from build123d import *

# Parameters (mm, degrees)
F0_W     = 134.5710605383
F0_H     = 126.8914490938
F0_W_2   = 120.110668242
F0_H_2   = 106.3882932067
F1_DEPTH = 50.8
F2_R     = 8.7009101407
F3_DEPTH = 508
F4_DEPTH = 25.4
F6_W     = 55.7228904217
F6_H     = 25.6094848633
F7_DEPTH = 584.2
F5_W     = 118.594430387
F5_H     = 112.178966403
F8_DEPTH = 508


with BuildPart() as f1:
    # F0 (on Top) → F1 (new body)
    with BuildSketch(Plane.XY):
        Rectangle(F0_W, F0_H)
        Rectangle(F0_W_2, F0_H_2, mode=Mode.SUBTRACT)
        Rectangle(F0_W_2, F0_H_2)
    extrude(amount=F1_DEPTH)

    # F2 (on face) → F3 (cut)
    with BuildSketch(Plane(origin=(-67.2855302691, 0, 0), x_dir=(0, -1, 0), z_dir=(-1, 0, 0))):
        with Locations((0, 22.9123719037)):
            Circle(F2_R)
    extrude(amount=-F3_DEPTH, mode=Mode.SUBTRACT)

    # F4 (add): a face of the model
    f4_faces = [f1.faces().sort_by_distance(p)[0] for p in [
        (0, 0, 50.8),
    ]]
    extrude(f4_faces, amount=F4_DEPTH)

    # F6 (on face) → F7 (cut)
    with BuildSketch(Plane(origin=(0, 63.4457245469, 0), x_dir=(-1, 0, 0), z_dir=(0, 1, 0))):
        with Locations((0.0916505232, 63.3952575684)):
            Rectangle(F6_W, F6_H)
    extrude(amount=-F7_DEPTH, mode=Mode.SUBTRACT)

    # F5 (on face) → F8 (cut)
    with BuildSketch(Plane.XY.offset(76.2)):
        Rectangle(F5_W, F5_H)
    extrude(amount=-F8_DEPTH, mode=Mode.SUBTRACT)


solid = f1.part
Geometry check sheet. Reference: the model listing, model coordinates, mm. A direction names the side the tool comes from. Round coordinates to 2 decimals unless told otherwise and drop trailing zeros. Order: outer loops, then holes, each group sorted by start corner. A loop starts at its lowest first (then second) coordinate and runs counter-clockwise, first axis right, second up. Notation, with made-up numbers: (59, 13) - (76, 13) arc R23 ccw to (76, 36) - close; hole circle Ø8 at (-22.5, -4). An arc over 180 degrees is marked (long way). One line per question, with ' | ' between items. Start each with the question number.
(1) Thickness scan on L1, parallel to X at y = 11, z = 43.5; L2, parallel to Z at x = -65.5, y = 0; L3, parallel to Y at x = 53.5, z = 7. Record the ranges inside material, lowest first. Write a range as [from, to].
(2) Release check for a two-part mould opening along Z. For faces 4 (the flat face through (0, 57, 0)), 5 (the cylindrical face through (-63.35, 1.89, 14.42)), 6 (the cylindrical face through (63.24, 1.89, 14.42)), 7 (the flat face through (-1, -56.089, 30)) record: released by +Z, released by -Z, zero draft, split by the parting line, or undercut.
(3) Sectioned sample at C-C on z = 66. Record the cut outline in (x, y).
(4) Sectioned sample at B-B on x = 29.5. Record the cut outline in (y, z), and give its area (3 significant figures).
(5) Depth check by flat-ended pin: pin 1 Ø10 at (x, z) = (26.5, 60) entering from -Y; pin 2 Ø15.5 at (y, z) = (0, 22.91) entering from -X; pin 3 Ø3.5 at (x, y) = (6.5, 60.5) entering from +Z. Enter the tip coordinate at first touch or a pass-through.
(6) Sectioned sample at A-A on y = 0. Record the cut outline in (x, z), and give its area (3 significant figures).
(7) Sectioned sample at D-D on z = 20. Record the cut outline in (x, y), and give its area (3 significant figures).
(8) Access from +Z, -Z, +X, -X, +Y, -Y to the whole of each face (thin tool, end or side, straight path). Record for faces 1 (the flat face through (-1, 56.089, 30)), 2 (the flat face through (61, 5, 76.2)), 3 (the flat face through (0, -60, 50.591)).
Conclusion:
1) L1: x = [-67.29, -59.3], [59.3, 67.29] | L2: z = [0, 14.21], [31.61, 76.2] | L3: y = [-63.45, -56.09], [56.09, 63.45]
2) face 4: released by -Z | face 5: undercut | face 6: undercut | face 7: zero draft
3) outline: (-67.29, -63.45) - (-27.95, -63.45) - (-27.95, -56.09) - (-59.3, -56.09) - (-59.3, 56.09) - (-27.95, 56.09) - (-27.95, 63.45) - (-67.29, 63.45) - close; (27.77, -63.45) - (67.29, -63.45) - (67.29, 63.45) - (27.77, 63.45) - (27.77, 56.09) - (59.3, 56.09) - (59.3, -56.09) - (27.77, -56.09) - close
4) outline: (-63.45, 0) - (-56.09, 0) - (-56.09, 76.2) - (-63.45, 76.2) - close; (56.09, 0) - (63.45, 0) - (63.45, 76.2) - (56.09, 76.2) - close | area: 1,120 mm2
5) pin 1: stops at y = -63.45 | pin 2: passes through | pin 3: stops at z = 50.59
6) outline: (-67.29, 0) - (-59.3, 0) - (-59.3, 14.21) - (-67.29, 14.21) - close; (-67.29, 31.61) - (-59.3, 31.61) - (-59.3, 76.2) - (-67.29, 76.2) - close; (59.3, 0) - (67.29, 0) - (67.29, 14.21) - (59.3, 14.21) - close; (59.3, 31.61) - (67.29, 31.61) - (67.29, 76.2) - (59.3, 76.2) - close | area: 939 mm2
7) outline: (-67.29, -63.45) - (67.29, -63.45) - (67.29, -8.2) - (59.3, -8.2) - (59.3, -56.09) - (-59.3, -56.09) - (-59.3, -8.2) - (-67.29, -8.2) - close; (-67.29, 8.2) - (-59.3, 8.2) - (-59.3, 56.09) - (59.3, 56.09) - (59.3, 8.2) - (67.29, 8.2) - (67.29, 63.45) - (-67.29, 63.45) - close | area: 3,510 mm2
8) face 1: +Z, -Z | face 2: +Z, +X, -X, +Y, -Y | face 3: +Z, +Y, -Y
